Read the model definition and answer for the solid it produces. Units are mm, in the model's axes. Face numbers are marked on the shaded views. A direction names the side the tool comes from. Coordinates: 2 decimals unless noted, no trailing zeros. Loops run counter-clockwise (first coordinate to the right, second up) from the corner with the lowest first, then second, coordinate; pieces in that order, holes last.
from build123d import *

# Parameters (mm, degrees)
F1_DEPTH = 20
F2_R     = 2.5
F3_DEPTH = 2.001
F4_R     = 1


with BuildPart() as f1:
    # F0 (on Front) → F1 (new body, symmetric)
    with BuildSketch(Plane.XZ):
        with BuildLine():
            Line((-92.5, 2), (-92.5, 0))
            Line((-92.5, 0), (-78, 0))
            ThreePointArc((-78, 0), (-75.171573, 1.171573), (-74, 4))
            Line((-74, 4), (-74, 46))
            ThreePointArc((-74, 46), (-73.414214, 47.414214), (-72, 48))
            Line((-72, 48), (0, 48))
            Line((0, 48), (72, 48))
            ThreePointArc((72, 48), (73.414214, 47.414214), (74, 46))
            Line((74, 46), (74, 4))
            ThreePointArc((74, 4), (75.171573, 1.171573), (78, 0))
            Line((78, 0), (92.5, 0))
            Line((92.5, 0), (92.5, 2))
            Line((92.5, 2), (78, 2))
            ThreePointArc((78, 2), (76.585786, 2.585786), (76, 4))
            Line((76, 4), (76, 46))
            ThreePointArc((76, 46), (74.828427, 48.828427), (72, 50))
            Line((72, 50), (0, 50))
            Line((0, 50), (-72, 50))
            ThreePointArc((-72, 50), (-74.828427, 48.828427), (-76, 46))
            Line((-76, 46), (-76, 4))
            ThreePointArc((-76, 4), (-76.585786, 2.585786), (-78, 2))
            Line((-78, 2), (-92.5, 2))
        make_face()
    extrude(amount=F1_DEPTH, both=True)

    # F2 (on face) → F3 (cut, through all)
    with BuildSketch(Plane.XY.offset(2)):
        with Locations((-85, 0)):
            Circle(F2_R)
        with Locations((85, 0)):
            Circle(F2_R)
    extrude(amount=-F3_DEPTH, mode=Mode.SUBTRACT)

    # F4
    f4_edges = [f1.edges().sort_by_distance(p)[0] for p in [
        (-92.5, -20, 1),
        (-92.5, 20, 1),
        (92.5, -20, 1),
        (92.5, 20, 1),
    ]]
    fillet(f4_edges, radius=F4_R)


solid = f1.part
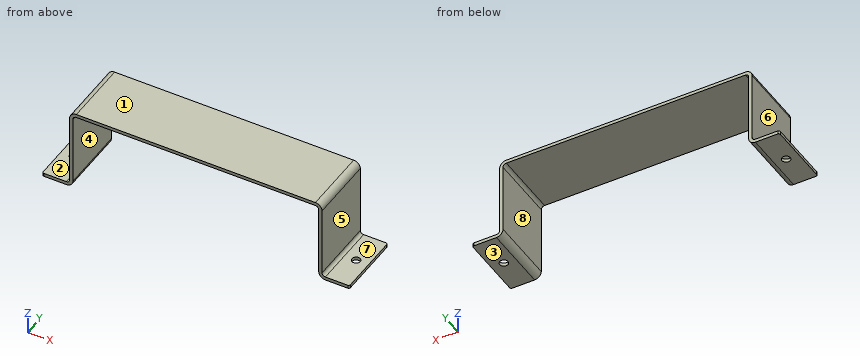
Q1. A cutting plane is placed at A-A (y = 0). Give the vertices of the cut face in (x, z), then the cut area to 3 significant figures.
Findings below:
outline: (-92.5, 0) - (-87.5, 0) - (-87.5, 2) - (-92.5, 2) - close; (-82.5, 0) - (-78, 0) arc R4 ccw to (-74, 4) - (-74, 46) arc R2 cw to (-72, 48) - (72, 48) arc R2 cw to (74, 46) - (74, 4) arc R4 ccw to (78, 0) - (82.5, 0) - (82.5, 2) - (78, 2) arc R2 cw to (76, 4) - (76, 46) arc R4 ccw to (72, 50) - (-72, 50) arc R4 ccw to (-76, 46) - (-76, 4) arc R2 cw to (-78, 2) - (-82.5, 2) - close; (87.5, 0) - (92.5, 0) - (92.5, 2) - (87.5, 2) - close
area: 532 mm2
Q2. A cutting plane is placed at D-D (y = 8). Give the vertices of the cut face in (x, z).
Findings below:
outline: (-92.5, 0) - (-78, 0) arc R4 ccw to (-74, 4) - (-74, 46) arc R2 cw to (-72, 48) - (72, 48) arc R2 cw to (74, 46) - (74, 4) arc R4 ccw to (78, 0) - (92.5, 0) - (92.5, 2) - (78, 2) arc R2 cw to (76, 4) - (76, 46) arc R4 ccw to (72, 50) - (-72, 50) arc R4 ccw to (-76, 46) - (-76, 4) arc R2 cw to (-78, 2) - (-92.5, 2) - close
Q3. Determine the mould class of the marked faces 6, 7 and 8 for opening direction X: +X half, -X half, draft (parallel to the pull), parting line (faces both ways), or undercut.
Findings below:
face 6: -X half
face 7: draft
face 8: undercut
Q4. Straight lines are drawn through the part: probe 1 along X at (y, z) = (1, 30); probe 2 along Y at (x, z) = (-85, 1.05); probe 3 along Z at (x, y) = (78, -17). For each, find the intervals that lie inside material, in ascending order.
Findings below:
probe 1: x = -76 to -74, 74 to 76
probe 2: y = -20 to -2.5, 2.5 to 20
probe 3: z = 0 to 2
Q5. Flat-ended cylindrical pins translate along their axes: pin 1 Ø1 at (y, z) = (5.5, 34.5) entering from -X; pin 2 Ø7 at (x, y) = (-83, -5) entering from +Z; pin 3 Ø1.5 at (x, y) = (-8, -14.5) entering from -Z. Find the tip coordinate at first contact, or state that the pin passes through.
Findings below:
pin 1: stops at x = -76
pin 2: stops at z = 2
pin 3: stops at z = 48
Q6. Which of the six approach directions +Z, -Z, +X, -X, +Y, -Y give full straight-line access (tool end or side, diameter ignored) to the marked faces 1, 2, 3, 4 and 5?
Findings below:
face 1: +Z, +X, -X, +Y, -Y
face 2: +Z, -X, +Y, -Y
face 3: -Z, +X, -X, +Y, -Y
face 4: -Z, +Y, -Y
face 5: +Z, +X, +Y, -Y
Q7. A cutting plane is placed at B-B (x = -85). Give the vertices of the cut face in (y, z).
Findings below:
outline: (-20, 0) - (-2.5, 0) - (-2.5, 2) - (-20, 2) - close; (2.5, 0) - (20, 0) - (20, 2) - (2.5, 2) - close
Q8. A cutting plane is placed at C-C (z = 22.5). Give the vertices of the cut face in (x, y).
Findings below:
outline: (-76, -20) - (-74, -20) - (-74, 20) - (-76, 20) - close; (74, -20) - (76, -20) - (76, 20) - (74, 20) - close
